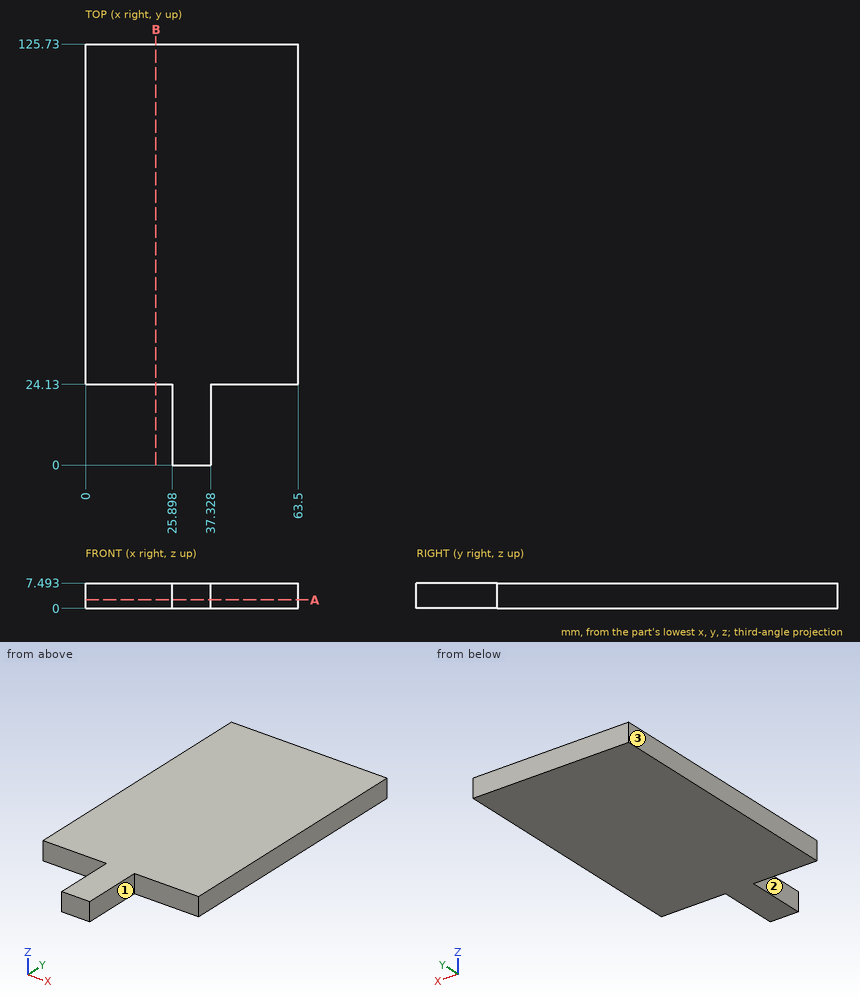
Study the drawing (mm; zero at the part's minimum x, y, z) and answer. A direction names the side the tool comes from. Coordinates: 2 decimals unless noted, no trailing zeros. Loops run counter-clockwise (first coordinate to the right, second up) from the corner with the lowest first, then second, coordinate; pieces in that order, holes last. Notation, with made-up numbers: (41, 67) -> (49, 67) arc R32 ccw to (49, 97) -> close; hole circle Ø7 at (66, 9.25). An arc over 180 degrees is marked (long way). Write item = value, one per line. Start each with the question number.
1) Given P1, Ø2, axis at y = 13.5, z = 5, coming from the +X side; P2, Ø3.5, axis at y = 12, z = 4, coming from the -X side; P3, Ø6, axis at x = 54.5, y = 53.5, coming from the -Z side; P4, Ø2, axis at x = 39, z = 5, coming from the -Y side, each flat-ended and moving along its own axis, determine where each tip first touches the part or whether it passes through.
2) Find the intervals of material crossed by L1, parallel to Y at x = 18.5, z = 4.75; L2, parallel to X at y = 19, z = 3, in increasing order. Write a range as from..to.
3) The part is cut by section A-A, the plane z = 2.5. Determine the outline of the cut face in (x, y).
4) The part is cut by section B-B, the plane x = 21. Determine the outline of the cut face in (y, z).
5) For the marked faces 1, 2 and 3, determine the directions among +Z, -Z, +X, -X, +Y, -Y from which every point of the face is accessible in a straight line to the end or side of a thin tool.
Result:
q1.P1 = 37.33
q1.P2 = 25.9
q1.P3 = 0
q1.P4 = 24.13
q2.L1 = 24.13..125.73
q2.L2 = 25.9..37.33
q3.outline = (0, 24.13) -> (25.9, 24.13) -> (25.9, 0) -> (37.33, 0) -> (37.33, 24.13) -> (63.5, 24.13) -> (63.5, 125.73) -> (0, 125.73) -> close
q4.outline = (24.13, 0) -> (125.73, 0) -> (125.73, 7.49) -> (24.13, 7.49) -> close
q5.face_1 = +Z, -Z, +X, -Y
q5.face_2 = +Z, -Z, -X, -Y
q5.face_3 = +Z, -Z, -X, +Y, -Y
